Geometry: see drawing. Coordinates: mm, zero at the bounding-box minimum. Coordinates: 2 decimals unless noted, no trailing zeros. Loops run counter-clockwise (first coordinate to the right, second up) from the corner with the lowest first, then second, coordinate; pieces in that order, holes last. Notation, with made-up numbers: (-27, -4) - (-19, -4) arc R30 ccw to (-19, 20) - close; hole circle Ø11 at (39, 64). An arc over 180 degrees is marked (long way). Write item = value, one per line. Start each with the question number.
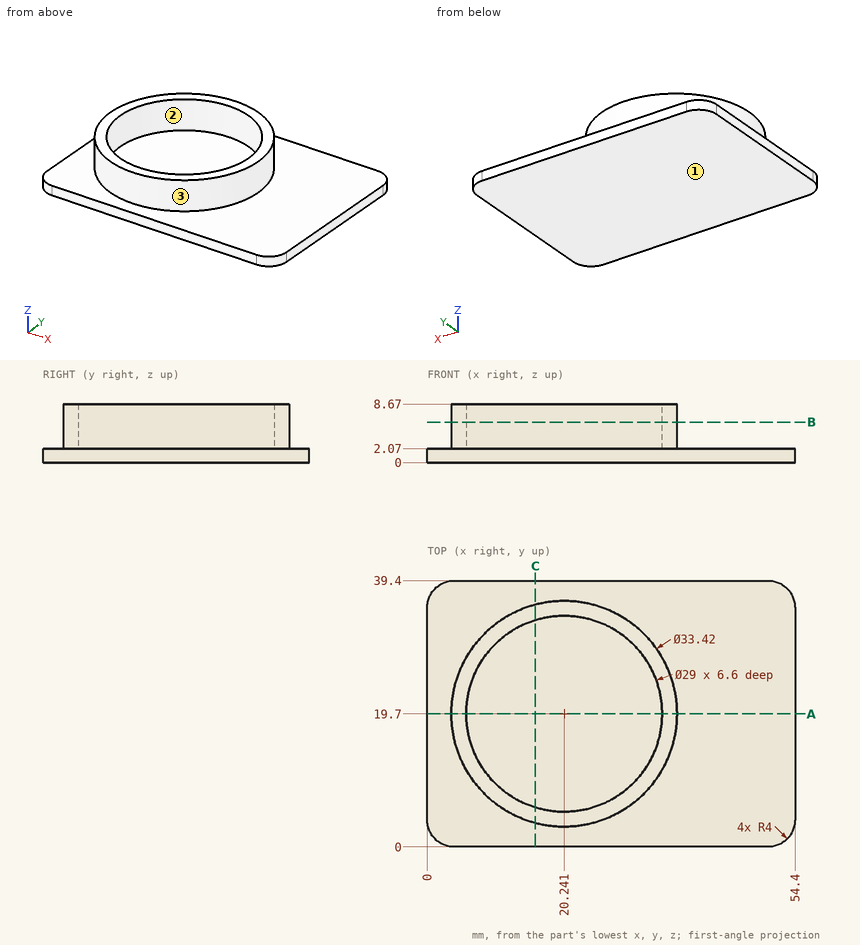
Item 1: Draft query along Y for the marked faces 1, 2 and 3. Return one class per face: released by +Y, released by -Y, zero draft, split by the parting line, or undercut.
Item 2: Cut plane B-B (z = 6). Return the cut outline in (x, y), then the cut area to 3 significant figures.
Item 3: First-contact query: pin 1 (8.5 mm diameter, centred on x = 18.5, y = 13, fed in from +Z); pin 2 (4 mm diameter, centred on x = 31.5, z = 6.5, fed in from +Y); pin 3 (1.5 mm diameter, centred on y = 7.5, z = 3, fed in from +X). Flat tips, straight axial feed; report the tip coordinate or a pass-through.
Item 4: Material intervals for L1, parallel to X at y = 19.7, z = 4.75; L2, parallel to Z at x = 15, y = 11; L3, parallel to Y at x = 22.5, z = 7.5, sorted ascending. Write a range as [from, to].
Item 5: Cut plane A-A (y = 19.7). Return the cut outline in (x, z).
Item 6: Cut plane C-C (x = 16). Return the cut outline in (y, z).
Responses:
q1.face_1 = zero draft
q1.face_2 = undercut
q1.face_3 = split by the parting line
q2.outline = circle Ø33.42 at (20.24, 19.7); hole circle Ø29 at (20.24, 19.7)
q2.area = 217 mm2
q3.pin_1 = 2.07
q3.pin_2 = 33.61
q3.pin_3 = 32.41
q4.L1 = [3.53, 5.74], [34.74, 36.95]
q4.L2 = [0, 2.07]
q4.L3 = [3.14, 5.38], [34.02, 36.26]
q5.outline = (0, 0) - (54.4, 0) - (54.4, 2.07) - (36.95, 2.07) - (36.95, 8.67) - (34.74, 8.67) - (34.74, 2.07) - (5.74, 2.07) - (5.74, 8.67) - (3.53, 8.67) - (3.53, 2.07) - (0, 2.07) - close
q6.outline = (0, 0) - (39.4, 0) - (39.4, 2.07) - (35.86, 2.07) - (35.86, 8.67) - (33.57, 8.67) - (33.57, 2.07) - (5.83, 2.07) - (5.83, 8.67) - (3.54, 8.67) - (3.54, 2.07) - (0, 2.07) - close
